Part print with two shaded views. Sizes in mm from the minimum x, y, z corner. A direction names the side the tool comes from. Coordinates: 2 decimals unless noted, no trailing zeros. Loops run counter-clockwise (first coordinate to the right, second up) from the corner with the lowest first, then second, coordinate; pieces in that order, holes last.
Item 1: Cut at B-B (x = 6). List the corners of the cut face in (y, z), and give its area (3 significant figures).
Item 2: Cut at A-A (z = 6). List the corners of the cut face in (x, y), and give its area (3 significant figures).
Item 3: Mould opens along X. For the marked faces 1, 2 and 3 say: released by +X, released by -X, zero draft, split by the parting line, or undercut.
Item 4: Drill centre lines: line 1 along Y through (x, z) = (10.5, 6.75); line 2 along Y through (x, z) = (9.25, 8.25); line 3 along X through (y, z) = (9, 6.5). Where is each one in solid material? Low to high.
Item 5: Cut at C-C (y = 2.25). List the corners of the cut face in (x, z).
Item 6: 3-axis set-ups, long thin cutter, end or side, ignore diameter. For the marked faces 4 and 5: which of +Z, -Z, +X, -X, +Y, -Y reach the whole face in a straight line?
Item 7: Cut at D-D (x = 3.5). List the corners of the cut face in (y, z), and give its area (3 significant figures).
Item 8: Flat gauge pins, fed straight in: pin 1 (1 mm diameter, centred on y = 9.5, z = 6.5, fed in from -X); pin 2 (1 mm diameter, centred on y = 19, z = 9, fed in from -X); pin 3 (3 mm diameter, centred on x = 5.5, y = 19, fed in from +Z). Where does each tip first touch, or does it go through?
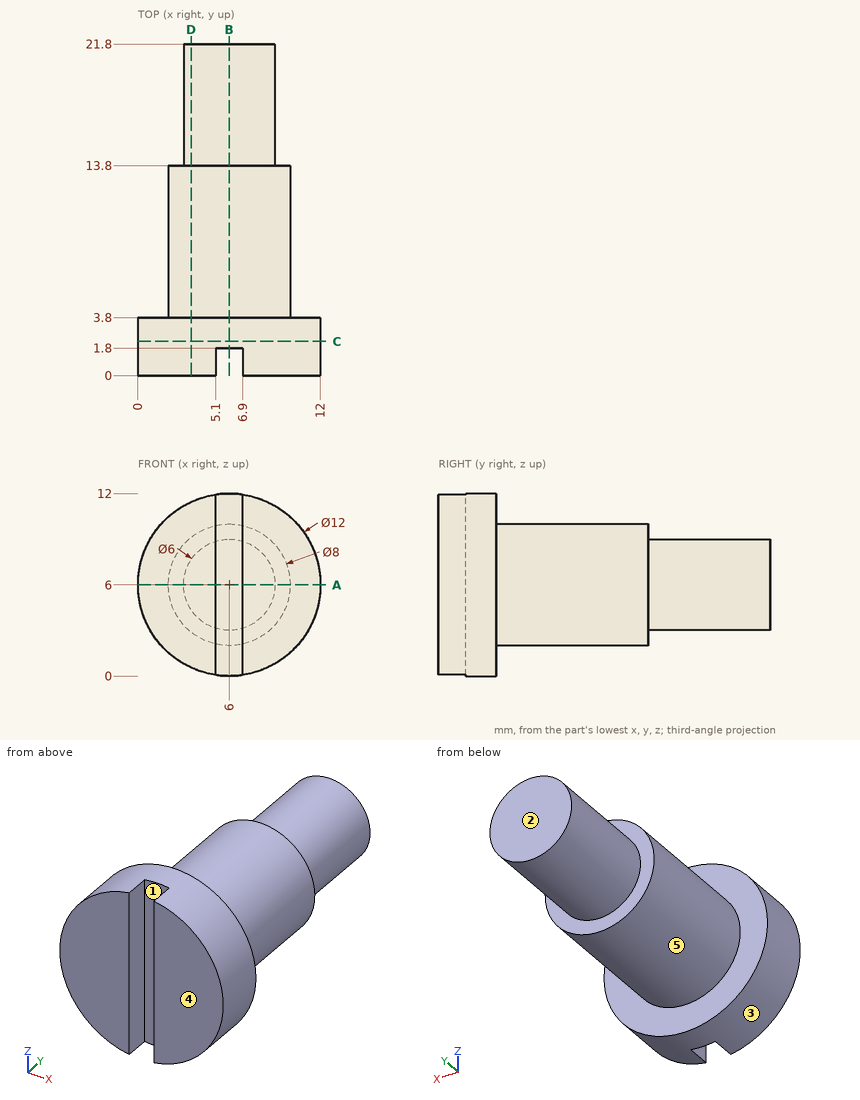
Filled sheet:
1. outline: (1.8, 0) - (3.8, 0) - (3.8, 2) - (13.8, 2) - (13.8, 3) - (21.8, 3) - (21.8, 9) - (13.8, 9) - (13.8, 10) - (3.8, 10) - (3.8, 12) - (1.8, 12) - close
1. area: 152 mm2
2. outline: (0, 0) - (5.1, 0) - (5.1, 1.8) - (6.9, 1.8) - (6.9, 0) - (12, 0) - (12, 3.8) - (10, 3.8) - (10, 13.8) - (9, 13.8) - (9, 21.8) - (3, 21.8) - (3, 13.8) - (2, 13.8) - (2, 3.8) - (0, 3.8) - close
2. area: 170 mm2
3. face 1: undercut
3. face 2: zero draft
3. face 3: split by the parting line
4. line 1: y = 0 to 3.8
4. line 2: y = 0 to 13.8
4. line 3: x = 2.03 to 9.97
5. outline: circle Ø12 at (6, 6)
6. face 4: +Z, -Z, +X, -X, -Y
6. face 5: +Y
7. outline: (0, 0.55) - (3.8, 0.55) - (3.8, 2.88) - (13.8, 2.88) - (13.8, 4.34) - (21.8, 4.34) - (21.8, 7.66) - (13.8, 7.66) - (13.8, 9.12) - (3.8, 9.12) - (3.8, 11.45) - (0, 11.45) - close
7. area: 130 mm2
8. pin 1: stops at x = 2
8. pin 2: stops at x = 4.34
8. pin 3: stops at z = 9
